The model under review builds one solid part; all positions refer to its coordinate system, in mm. Face numbers are marked on the shaded views. A direction names the side the tool comes from. Give positions to 0.01 mm unless a question says otherwise; leave off trailing zeros. Order: outer loops, then holes, each group sorted by start corner. A loop starts at its lowest first (then second) coordinate and runs counter-clockwise, first axis right, second up. Notation, with made-up numbers: (51, 86) - (77, 86) arc R20 ccw to (77, 96) - close; hole circle Ø11 at (84.5, 62). An arc over 180 degrees is marked (long way). Use a Markdown table: item, result. Add a question column.
```python
from build123d import *

# Parameters (mm, degrees)
SKETCH2_W                    = 170
SKETCH2_H                    = 110
BASE_FLANGE1_DEPTH           = 8
EDGE_FLANGE1_STRIP_W         = 52
EDGE_FLANGE1_STRIP_H         = 8
EDGE_FLANGE1_STRIP_CUT_DEPTH = 110
EDGE_FLANGE1_DEPTH           = 110


# Sheet-metal steps are written as plain solids
with BuildPart() as part:
    # Sketch2 → Base-Flange1 (new body)
    with BuildSketch(Plane(origin=(0, 0, 0), x_dir=(1, 0, 0), z_dir=(0, 1, 0))):
        Rectangle(SKETCH2_W, SKETCH2_H)
    extrude(amount=-BASE_FLANGE1_DEPTH)

    # Edge-Flange1 strip (across the edge) → Edge-Flange1 strip cut (cut)
    with BuildSketch(Plane(origin=(85, 0, 55), x_dir=(-1, 0, 0), z_dir=(0, 0, -1))):
        with Locations((-8, -4)):
            Rectangle(EDGE_FLANGE1_STRIP_W, EDGE_FLANGE1_STRIP_H)
    extrude(amount=EDGE_FLANGE1_STRIP_CUT_DEPTH, mode=Mode.SUBTRACT)

    # Edge-Flange1 section (across the edge) → Edge-Flange1 (add)
    with BuildSketch(Plane(origin=(85, 0, 55), x_dir=(-1, 0, 0), z_dir=(0, 0, -1))):
        with BuildLine():
            Line((0, 10), (0, 42))
            Line((0, 42), (8, 42))
            Line((8, 42), (8, 10))
            ThreePointArc((8, 10), (10.928932188, 2.928932188), (18, 0))
            Line((18, 0), (18, -8))
            ThreePointArc((18, -8), (5.272077939, -2.727922061), (0, 10))
        make_face()
    extrude(amount=EDGE_FLANGE1_DEPTH)

    # Mirror1: part across plane


with BuildPart() as part_1:
    add(part.part)
    add(part.part.mirror(Plane(origin=(-85, -8, 55), x_dir=(0, 0, 1), z_dir=(-1, 0, 0))))


solid = part_1.part
```
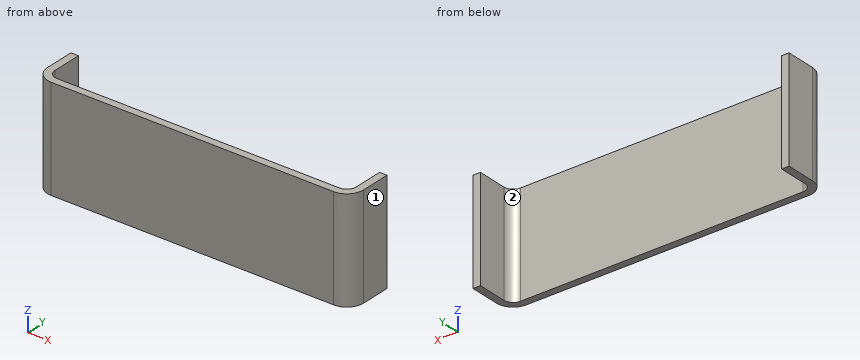
Q1. Clearance check with a flat-ended pin moving along its axis: P1, Ø4, axis at x = -50, z = -35.5, coming from the +Y side. State where the tip first meets the part, or that it passes through.
Q2. Wall thickness on probe 1 along X at (y, z) = (10, -39); probe 2 along Y at (x, z) = (61, -2.5); probe 3 along X at (y, z) = (5.5, -31): over which ranges is each line inside the solid? List them lowest first.
Q3. Machinability: for the marked faces 1 and 2, which of the approach directions +Z, -Z, +X, -X, +Y, -Y give a long, thin tool a straight path to every point of the face, cutting with its end or side? Answer none if there is none.
Q4. We need section B-B (z = -29.5). Write out the cut boundary in (x, y), plus the area to 3 significant figures.
Q5. We need section A-A (y = 14). Write out the cut boundary in (x, z), plus the area to 3 significant figures.
Q6. We need section C-C (x = -164). Write out the cut boundary in (y, z).
Here are the results:
| question | item | result |
|---|---|---|
| 1 | P1 | y = 0 |
| 2 | probe 1 | -255 to -247, 77 to 85 |
| 2 | probe 2 | -8 to 0 |
| 2 | probe 3 | -254.43 to -245.93, 75.93 to 84.43 |
| 3 | face 1 | +Z, -Z, +X, +Y, -Y |
| 3 | face 2 | +Z, -Z, +Y |
| 4 | outline | (-255, 10) arc R18 ccw to (-237, -8) - (67, -8) arc R18 ccw to (85, 10) - (85, 42) - (77, 42) - (77, 10) arc R10 cw to (67, 0) - (-237, 0) arc R10 cw to (-247, 10) - (-247, 42) - (-255, 42) - close |
| 4 | area | 3,300 mm2 |
| 5 | outline | (-255, -55) - (-247, -55) - (-247, 55) - (-255, 55) - close; (77, -55) - (85, -55) - (85, 55) - (77, 55) - close |
| 5 | area | 1,760 mm2 |
| 6 | outline | (-8, -55) - (0, -55) - (0, 55) - (-8, 55) - close |
